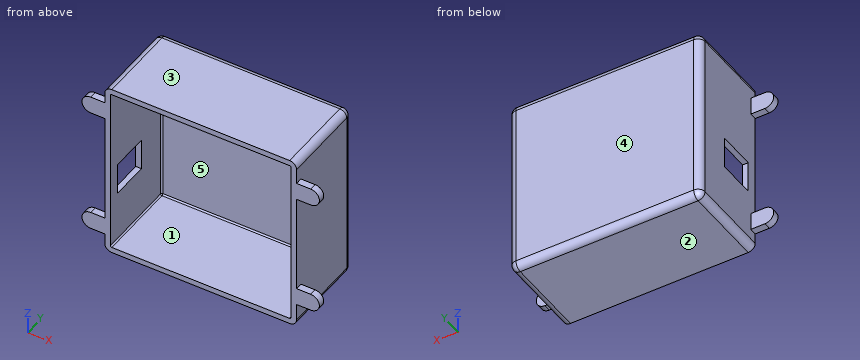
from build123d import *

# Parameters (mm, degrees)
SKETCH1_W           = 48.3
SKETCH1_H           = 45
BOSS_EXTRUDE1_DEPTH = 25
FILLET1_R           = 2
SHELL1_T            = -1.6
BOSS_EXTRUDE2_DEPTH = 2
SKETCH2_W           = 9
SKETCH2_H           = 11
CUT_EXTRUDE1_DEPTH  = 70.553217036


with BuildPart() as part:
    # Sketch1 → Boss-Extrude1 (new body)
    # profile 1 of 2: a face of its own
    with BuildSketch(Plane(origin=(0, 0, 0), x_dir=(1, 0, 0), z_dir=(0, 1, 0))):
        Polygon((27.35, 20.7), (27.35, 25.7), (-27.35, 25.7), (-27.35, 20.7), (-27.35, 15.7), (-27.35, -15.7), (-27.35, -20.7), (-27.35, -25.7), (27.35, -25.7), (27.35, -19.351788551), (27.35, -14.351788551), (27.35, 13.848211449), (27.35, 18.848211449), align=None)
        Rectangle(SKETCH1_W, SKETCH1_H, mode=Mode.SUBTRACT)
    # profile 2 of 2: a face of its own
    with BuildSketch(Plane(origin=(0, 0, 0), x_dir=(1, 0, 0), z_dir=(0, 1, 0))):
        Rectangle(SKETCH1_W, SKETCH1_H)
    extrude(amount=BOSS_EXTRUDE1_DEPTH)

    # Fillet1
    fillet1_edges = [part.edges().sort_by_distance(p)[0] for p in [
        (-27.35, 25, 0),
        (0, 25, 25.7),
        (27.35, 25, 0),
        (0, 25, -25.7),
        (27.35, 12.5, 25.7),
        (-27.35, 12.5, 25.7),
        (-27.35, 12.5, -25.7),
        (27.35, 12.5, -25.7),
    ]]
    fillet(fillet1_edges, radius=FILLET1_R)

    # Shell1
    shell1_openings = [part.faces().sort_by_distance(p)[0] for p in [
        (0, 0, 0),
    ]]
    offset(amount=SHELL1_T, openings=shell1_openings, kind=Kind.INTERSECTION)

    # Sketch1_3 → Boss-Extrude2 (add)
    with BuildSketch(Plane(origin=(0, 0, 0), x_dir=(1, 0, 0), z_dir=(0, 1, 0))):
        with BuildLine():
            Line((31.35, 18.848211449), (27.35, 18.848211449))
            Line((27.35, 18.848211449), (27.35, 13.848211449))
            Line((27.35, 13.848211449), (31.35, 13.848211449))
            ThreePointArc((31.35, 13.848211449), (33.85, 16.348211449), (31.35, 18.848211449))
        make_face()
        with BuildLine():
            Line((-27.35, 15.7), (-27.35, 20.7))
            Line((-27.35, 20.7), (-31.35, 20.7))
            ThreePointArc((-31.35, 20.7), (-33.85, 18.2), (-31.35, 15.7))
            Line((-31.35, 15.7), (-27.35, 15.7))
        make_face()
        with BuildLine():
            Line((31.35, -14.351788551), (27.35, -14.351788551))
            Line((27.35, -14.351788551), (27.35, -19.351788551))
            Line((27.35, -19.351788551), (31.35, -19.351788551))
            ThreePointArc((31.35, -19.351788551), (33.85, -16.851788551), (31.35, -14.351788551))
        make_face()
        with BuildLine():
            Line((-27.35, -20.7), (-27.35, -15.7))
            Line((-27.35, -15.7), (-31.35, -15.7))
            ThreePointArc((-31.35, -15.7), (-33.85, -18.2), (-31.35, -20.7))
            Line((-31.35, -20.7), (-27.35, -20.7))
        make_face()
    extrude(amount=BOSS_EXTRUDE2_DEPTH)

    # Sketch2 → Cut-Extrude1 (cut, through all)
    with BuildSketch(Plane(origin=(-25.75, 0, 0), x_dir=(0, 0, -1), z_dir=(1, 0, 0))):
        with Locations((5, 8.7)):
            Rectangle(SKETCH2_W, SKETCH2_H)
    extrude(amount=-CUT_EXTRUDE1_DEPTH, mode=Mode.SUBTRACT)


solid = part.part
Verification items for the finished model (mm, model axes). Face numbers are marked on the shaded views. A direction names the side the tool comes from. Give positions to 0.01 mm unless a question says otherwise; leave off trailing zeros. Loops run counter-clockwise (first coordinate to the right, second up) from the corner with the lowest first, then second, coordinate; pieces in that order, holes last. Notation, with made-up numbers: (30.25, 49) - (83.25, 49) arc R21 cw to (83.25, 76) - close; hole circle Ø1 at (83.25, 8.25). An arc over 180 degrees is marked (long way). Write item = value, one per line. Start each with the question number.
Q1. Cross-section at B-B, the plane z = -8.5. Enter the section's corners in (x, y).
Q2. Mould release check, pull along Z, two halves, no side actions. Record for the marked faces 3, 4 and 5: released by +Z, released by -Z, zero draft, split by the parting line, or undercut.
Q3. Depth check by flat-ended pin: P1, Ø4, axis at y = 17, z = -6, coming from the -X side; P2, Ø5, axis at y = 18.5, z = 10, coming from the +X side; P3, Ø1.6, axis at x = -30, y = 0.5, coming from the -Z side. Enter the tip coordinate at first touch or a pass-through.
Q4. Cross-section at C-C, the plane x = 17. Enter the section's corners in (y, z), and give its area (3 significant figures).
Q5. Cross-section at D-D, the plane y = 8. Enter the section's corners in (x, z).
Q6. Tool access check on the marked faces 1 and 2. Record the directions out of +Z, -Z, +X, -X, +Y, -Y that give a thin tool (end or side, any length) a straight path to the whole face; none if there is none.
Q7. Thickness scan on line 1 (Z direction, x = 23, y = 11.25); line 2 (X direction, y = 20.5, z = 22); line 3 (Y direction, x = -1.5, z = 12.5). Record the ranges inside material, lowest first.
Q8. Cross-section at A-A, the plane y = 21. Enter the section's corners in (x, z).
Answer key:
q1.outline = (-27.35, 0) - (-25.75, 0) - (-25.75, 3.2) - (-27.35, 3.2) - close; (-27.35, 14.2) - (-25.75, 14.2) - (-25.75, 23) arc R0.4 cw to (-25.35, 23.4) - (25.35, 23.4) arc R0.4 cw to (25.75, 23) - (25.75, 0) - (27.35, 0) - (27.35, 23) arc R2 ccw to (25.35, 25) - (-25.35, 25) arc R2 ccw to (-27.35, 23) - close
q2.face_3 = released by +Z
q2.face_4 = zero draft
q2.face_5 = undercut
q3.P1 = -27.35
q3.P2 = 27.35
q3.P3 = -20.7
q4.outline = (0, -25.7) - (23, -25.7) arc R2 ccw to (25, -23.7) - (25, 23.7) arc R2 ccw to (23, 25.7) - (0, 25.7) - (0, 24.1) - (23, 24.1) arc R0.4 cw to (23.4, 23.7) - (23.4, -23.7) arc R0.4 cw to (23, -24.1) - (0, -24.1) - close
q4.area = 155 mm^2
q5.outline = (-27.35, -23.7) arc R2 ccw to (-25.35, -25.7) - (25.35, -25.7) arc R2 ccw to (27.35, -23.7) - (27.35, 23.7) arc R2 ccw to (25.35, 25.7) - (-25.35, 25.7) arc R2 ccw to (-27.35, 23.7) - (-27.35, -0.5) - (-25.75, -0.5) - (-25.75, 23.7) arc R0.4 cw to (-25.35, 24.1) - (25.35, 24.1) arc R0.4 cw to (25.75, 23.7) - (25.75, -23.7) arc R0.4 cw to (25.35, -24.1) - (-25.35, -24.1) arc R0.4 cw to (-25.75, -23.7) - (-25.75, -9.5) - (-27.35, -9.5) - close
q6.face_1 = -Y
q6.face_2 = -Z, +X, -X, +Y, -Y
q7.line_1 = -25.7 to -24.1, 24.1 to 25.7
q7.line_2 = -27.35 to -25.75, 25.75 to 27.35
q7.line_3 = 23.4 to 25
q8.outline = (-27.35, -23.7) arc R2 ccw to (-25.35, -25.7) - (25.35, -25.7) arc R2 ccw to (27.35, -23.7) - (27.35, 23.7) arc R2 ccw to (25.35, 25.7) - (-25.35, 25.7) arc R2 ccw to (-27.35, 23.7) - close; hole (-25.75, -23.7) arc R0.4 ccw to (-25.35, -24.1) - (25.35, -24.1) arc R0.4 ccw to (25.75, -23.7) - (25.75, 23.7) arc R0.4 ccw to (25.35, 24.1) - (-25.35, 24.1) arc R0.4 ccw to (-25.75, 23.7) - close
